The listing builds one solid part. Answer for the finished solid, in the listing's coordinates (mm). Face numbers are marked on the shaded views. A direction names the side the tool comes from. Coordinates: 2 decimals unless noted, no trailing zeros. Loops run counter-clockwise (first coordinate to the right, second up) from the corner with the lowest first, then second, coordinate; pieces in that order, holes last. Notation, with made-up numbers: (-8, 57.25) - (20, 57.25) arc R25 ccw to (20, 71.25) - close; hole circle Ø10 at (24.5, 7.5). An arc over 180 degrees is marked (long way). Put each result on its own line as item: value.
```python
from build123d import *

# Parameters (mm, degrees)
BOSS_EXTRUDE1_DEPTH = 10
FILLET1_R           = 1
SKETCH3_R           = 1.75
CUT_EXTRUDE1_DEPTH  = 1.8


with BuildPart() as part:
    # Sketch2 → Boss-Extrude1 (new body)
    with BuildSketch(Plane.XY):
        with BuildLine():
            Line((0, 0), (10.253572501, 0))
            ThreePointArc((10.253572501, 0), (12.826786251, 3.373213749), (16.2, 0.8))
            Line((16.2, 0.8), (17, 0.8))
            ThreePointArc((17, 0.8), (13.226786251, 4.194356599), (9.453572501, 0.8))
            Line((9.453572501, 0.8), (0, 0.8))
            Line((0, 0.8), (0, 0))
        make_face()
    extrude(amount=BOSS_EXTRUDE1_DEPTH)

    # Fillet1
    fillet1_edges = [part.edges().sort_by_distance(p)[0] for p in [
        (9.453572501, 0.8, 5),
        (10.253572501, 0, 5),
    ]]
    fillet(fillet1_edges, radius=FILLET1_R)

    # Sketch3 → Cut-Extrude1 (cut, through all)
    with BuildSketch(Plane(origin=(0, 0.8, 0), x_dir=(1, 0, 0), z_dir=(0, 1, 0))):
        with Locations((5.713393125, -5)):
            Circle(SKETCH3_R)
    extrude(amount=-CUT_EXTRUDE1_DEPTH, mode=Mode.SUBTRACT)


solid = part.part
```
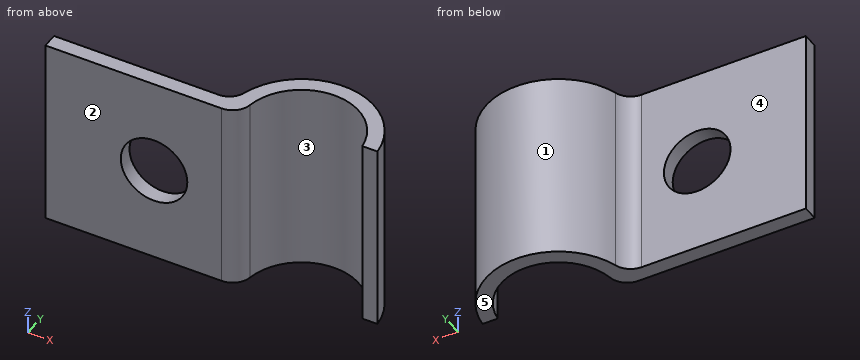
1) The part is cut by section C-C (y = 2.05). Give the vertices of the cut face in (x, z), and give its area (3 significant figures).
Found:
outline: (9.81, 0) - (10.72, 0) - (10.72, 10) - (9.81, 10) - close; (15.73, 0) - (16.64, 0) - (16.64, 10) - (15.73, 10) - close
area: 18.2 mm^2
2) The part is cut by section D-D (z = 7.25). Give the vertices of the cut face in (x, y), and give its area (3 significant figures).
Found:
outline: (0, 0) - (9.27, 0) arc R1 ccw to (10.26, 0.85) arc R3 cw to (16.2, 0.8) - (17, 0.8) arc R3.79 ccw to (9.6, 1.51) arc R1 cw to (8.64, 0.8) - (0, 0.8) - close
area: 16.0 mm^2
3) The part is cut by section A-A (z = 5). Give the vertices of the cut face in (x, y).
Found:
outline: (0, 0) - (3.96, 0) - (3.96, 0.8) - (0, 0.8) - close; (7.46, 0) - (9.27, 0) arc R1 ccw to (10.26, 0.85) arc R3 cw to (16.2, 0.8) - (17, 0.8) arc R3.79 ccw to (9.6, 1.51) arc R1 cw to (8.64, 0.8) - (7.46, 0.8) - close
4) For the marked faces 4 and 5, determine the directions among +Z, -Z, +X, -X, +Y, -Y from which every point of the face is accessible in a straight line to the end or side of a thin tool.
Found:
face 4: +Z, -Z, -X, +Y
face 5: -Z, +X, -X, +Y, -Y
5) Straight lines are drawn through the part: L1, parallel to Y at x = 6, z = 7.5; L2, parallel to X at y = 2.85, z = 1.75; L3, parallel to X at y = 2.7, z = 4. For each, find the intervals that lie inside material, in ascending order. Write a range as [from, to].
Found:
L1: y = [0, 0.8]
L2: x = [10.33, 11.5], [14.96, 16.12]
L3: x = [10.21, 11.3], [15.15, 16.24]
6) The part is cut by section B-B (x = 5). Give the vertices of the cut face in (y, z), and give its area (3 significant figures).
Found:
outline: (0, 0) - (0.8, 0) - (0.8, 3.4) - (0, 3.4) - close; (0, 6.6) - (0.8, 6.6) - (0.8, 10) - (0, 10) - close
area: 5.44 mm^2
7) For a pull along X with two mould halves and no side action, classify the marked faces 1, 2 and 3 as pulls with the +X half, pulls with the -X half, needs draft (parallel to the pull), parting line crosses it, or undercut.
Found:
face 1: parting line crosses it
face 2: needs draft
face 3: undercut
8) Each of these flat-tipped pins is pushed along its axis until it touches: pin 1 (1 mm diameter, centred on x = 7, y = 0.5, fed in from -Z); pin 2 (2 mm diameter, centred on x = 5.71, z = 5, fed in from +Y); pin 3 (4.5 mm diameter, centred on x = 4.5, z = 6.5, fed in from +Y); pin 4 (0.9 mm diameter, centred on x = 16.5, z = 5, fed in from -Y). Where does it stop, or does it pass through?
Found:
pin 1: stops at z = 0
pin 2: passes through
pin 3: stops at y = 0.8
pin 4: stops at y = 0.8
